Input: part model. Units: mm. Frame: model coordinates. Face numbers are marked on the shaded views. A direction names the side the tool comes from. Coordinates: 2 decimals unless noted, no trailing zeros. Order: outer loops, then holes, each group sorted by start corner. A loop starts at its lowest first (then second) coordinate and runs counter-clockwise, first axis right, second up. Notation, with made-up numbers: (21.25, -20.75) - (79.25, -20.75) arc R21 cw to (79.25, 1.25) - close; hole circle Ø1 at (-23, 76.5). An arc over 180 degrees is marked (long way). Answer as CSV lines item,"result". Start each with the question number.
Item 1: Section A-A (x = 0). Output: boundary loops of the cut face in (y, z), and give its area (3 significant figures).
Item 2: Section B-B (z = -1). Output: boundary loops of the cut face in (x, y).
Item 3: Section C-C (y = 4.75). Output: boundary loops of the cut face in (x, z).
Item 4: Section D-D (x = 4.5). Output: boundary loops of the cut face in (y, z), and give its area (3 significant figures).
Item 5: Draft query along Z for the marked faces 1, 2, 3 and 4. Return one class per face: +Z half, -Z half, draft (parallel to the pull), parting line (faces both ways), or undercut.
Item 6: Access query for the marked faces 5 and 6. Directions: +Z, -Z, +X, -X, +Y, -Y. A direction counts if a zero-diameter tool reaches every point of the face in a straight line with its end or side. Return the directions, or none.
Item 7: Material intervals for line 1 along Y through (x, z) = (4, -2.5); line 2 along Y through (x, z) = (-1.5, -1.75); line 3 along Z through (x, y) = (-2.25, -2), sorted ascending.
Item 8: First-contact query: pin 1 (5 mm diameter, centred on x = -2.5, y = 17, fed in from -Z); pin 2 (5.5 mm diameter, centred on x = 1.5, z = 0.5, fed in from -Y); pin 3 (1 mm diameter, centred on x = 3.5, z = 2, fed in from +Y); pin 4 (2 mm diameter, centred on x = 2, y = 7, fed in from +Z). Flat tips, straight axial feed; report the tip coordinate or a pass-through.
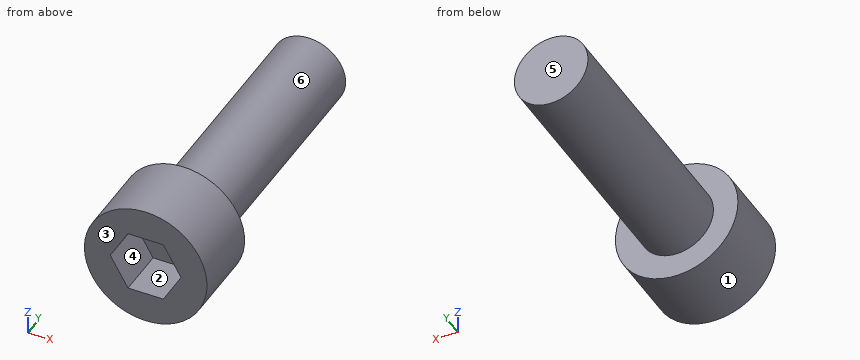
Autodesk Inventor part; units mm, degrees
ref_plane "YZ Plane" through (0, 0, 0) normal (1, 0, 0) x (0, 1, 0)
ref_plane "XZ Plane" through (0, 0, 0) normal (0, 1, 0) x (-1, 0, 0)
ref_plane "XY Plane" through (0, 0, 0) normal (0, 0, 1) x (1, 0, 0)
sketch "Szkic1" plane through (0, 0, 0) normal (0, 1, 0) x (-1, 0, 0)
  circle A0 centre (0, 0) radius 5
  line L0 (1.4434, 2.5) -> (2.8868, 0)
  line L1 (2.8868, 0) -> (1.4434, -2.5)
  line L2 (1.4434, -2.5) -> (-1.4434, -2.5)
  line L3 (-1.4434, -2.5) -> (-2.8868, 0)
  line L4 (-2.8868, 0) -> (-1.4434, 2.5)
  line L5 (-1.4434, 2.5) -> (1.4434, 2.5)
  circle A1 centre (0, 0) radius 3
  dimension "d0" = 10
  dimension "d1" = 5
  dimension "d2" = 6
extrude "Wyciągnięcie proste1" add sketch "Szkic1" along normal blind 2 contours A0 | L0 L1 L2 L3 L4 L5 | A1
extrude "Wyciągnięcie proste2" add sketch "Szkic1" against normal blind 4 contours A0 | A1
sketch "Szkic2" plane through (0, 2, 0) normal (0, 1, 0) x (1, 0, 0)
  circle A0 centre (0, 0) radius 3
  dimension "d7" = 6
extrude "Wyciągnięcie proste3" add sketch "Szkic2" along normal blind 20
thread "Gwint1"
properties part number "M6x20"
Determined:
1,outline,"(-4, -5) - (2, -5) - (2, -3) - (22, -3) - (22, 3) - (2, 3) - (2, 5) - (-4, 5) - (-4, 2.5) - (0, 2.5) - (0, -2.5) - (-4, -2.5) - close"
1,area,"160 mm^2"
2,outline,"(-4.9, -4) - (-2.31, -4) - (-2.31, 0) - (2.31, 0) - (2.31, -4) - (4.9, -4) - (4.9, 2) - (2.83, 2) - (2.83, 22) - (-2.83, 22) - (-2.83, 2) - (-4.9, 2) - close"
3,outline,"circle Ø6 at (0, 0)"
4,outline,"(-4, -2.18) - (2, -2.18) - (2, 2.18) - (-4, 2.18) - close"
4,area,"26.2 mm^2"
5,face 1,"parting line"
5,face 2,"undercut"
5,face 3,"draft"
5,face 4,"undercut"
6,face 5,"+Z, -Z, +X, -X, +Y"
6,face 6,"+Y"
7,line 1,"y = -4 to 2"
7,line 2,"y = 0 to 22"
7,line 3,"z = -4.47 to -1.1, 1.1 to 4.47"
8,pin 1,"stops at z = -3"
8,pin 2,"stops at y = -4"
8,pin 3,"stops at y = 2"
8,pin 4,"stops at z = 2.83"
